Build history of the part. All positions in model axes, mm. Face numbers are marked on the shaded views. A direction names the side the tool comes from. Round coordinates to 2 decimals unless told otherwise and drop trailing zeros. Write each loop counter-clockwise with the first axis right and the second up, starting at its lowest first coordinate (ties: lowest second). Pieces come first, ordered by that corner, then holes. Notation, with made-up numbers: (-3.75, 23.5) - (11.25, 23.5) arc R22 ccw to (11.25, 42.5) - close; hole circle Ø11 at (-12.75, -8). An arc over 180 degrees is marked (long way). One line per question, with ' | ' between items.
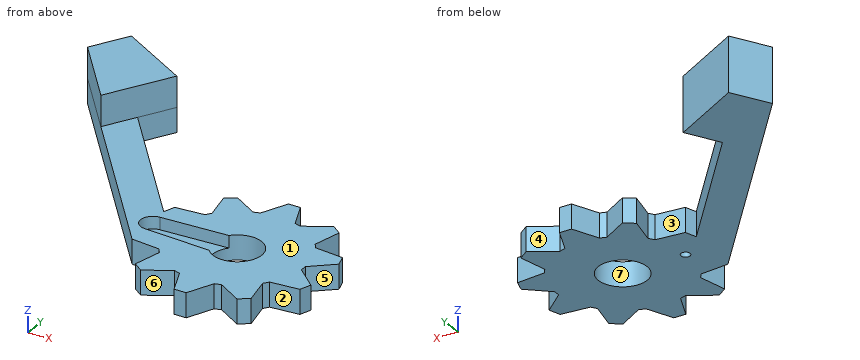
from build123d import *

# Parameters (mm, degrees)
SKETCH1_R           = 3.5
BOSS_EXTRUDE1_DEPTH = 4
BOSS_EXTRUDE2_DEPTH = 4
CUT_EXTRUDE1_DEPTH  = 2
SKETCH5_R           = 0.75
CUT_EXTRUDE2_DEPTH  = 59.571601855
SKETCH6_R           = 4
CUT_EXTRUDE3_DEPTH  = 10
BOSS_EXTRUDE3_DEPTH = 5


with BuildPart() as part:
    # Sketch1 → Boss-Extrude1 (new body)
    with BuildSketch(Plane.XY):
        with BuildLine():
            Line((-1, 15), (1, 15))
            Line((1, 15), (2.890622598, 10.613401952))
            ThreePointArc((2.890622598, 10.613401952), (3.399186938, 10.461621679), (3.899838338, 10.28548788))
            Line((3.899838338, 10.28548788), (8.00776179, 12.723040168))
            Line((8.00776179, 12.723040168), (9.625795779, 11.547469663))
            Line((9.625795779, 11.547469663), (8.57696395, 6.887357214))
            ThreePointArc((8.57696395, 6.887357214), (8.899186938, 6.465637775), (9.200693579, 6.02886703))
            Line((9.200693579, 6.02886703), (13.95683075, 5.586311432))
            Line((13.95683075, 5.586311432), (14.574864739, 3.684198399))
            Line((14.574864739, 3.684198399), (10.987196594, 0.530576113))
            ThreePointArc((10.987196594, 0.530576113), (11, 0), (10.987196594, -0.530576113))
            Line((10.987196594, -0.530576113), (14.574864739, -3.684198399))
            Line((14.574864739, -3.684198399), (13.95683075, -5.586311432))
            Line((13.95683075, -5.586311432), (9.200693579, -6.02886703))
            ThreePointArc((9.200693579, -6.02886703), (8.899186938, -6.465637775), (8.57696395, -6.887357214))
            Line((8.57696395, -6.887357214), (9.625795779, -11.547469663))
            Line((9.625795779, -11.547469663), (8.00776179, -12.723040168))
            Line((8.00776179, -12.723040168), (3.899838338, -10.28548788))
            ThreePointArc((3.899838338, -10.28548788), (3.399186938, -10.461621679), (2.890622598, -10.613401952))
            Line((2.890622598, -10.613401952), (1, -15))
            Line((1, -15), (-1, -15))
            Line((-1, -15), (-2.890622598, -10.613401952))
            ThreePointArc((-2.890622598, -10.613401952), (-3.399186938, -10.461621679), (-3.899838338, -10.28548788))
            Line((-3.899838338, -10.28548788), (-8.00776179, -12.723040168))
            Line((-8.00776179, -12.723040168), (-9.625795779, -11.547469663))
            Line((-9.625795779, -11.547469663), (-8.57696395, -6.887357214))
            ThreePointArc((-8.57696395, -6.887357214), (-8.899186938, -6.465637775), (-9.200693579, -6.02886703))
            Line((-9.200693579, -6.02886703), (-13.95683075, -5.586311432))
            Line((-13.95683075, -5.586311432), (-14.574864739, -3.684198399))
            Line((-14.574864739, -3.684198399), (-10.987196594, -0.530576113))
            ThreePointArc((-10.987196594, -0.530576113), (-11, 0), (-10.987196594, 0.530576113))
            Line((-10.987196594, 0.530576113), (-14.574864739, 3.684198399))
            Line((-14.574864739, 3.684198399), (-13.95683075, 5.586311432))
            Line((-13.95683075, 5.586311432), (-9.200693579, 6.02886703))
            ThreePointArc((-9.200693579, 6.02886703), (-8.899186938, 6.465637775), (-8.57696395, 6.887357214))
            Line((-8.57696395, 6.887357214), (-9.625795779, 11.547469663))
            Line((-9.625795779, 11.547469663), (-8.00776179, 12.723040168))
            Line((-8.00776179, 12.723040168), (-3.899838338, 10.28548788))
            ThreePointArc((-3.899838338, 10.28548788), (-3.399186938, 10.461621679), (-2.890622598, 10.613401952))
            Line((-2.890622598, 10.613401952), (-1, 15))
        make_face()
        Circle(SKETCH1_R, mode=Mode.SUBTRACT)
    extrude(amount=-BOSS_EXTRUDE1_DEPTH)

    # Sketch3 → Boss-Extrude2 (add)
    with BuildSketch(Plane.XY):
        Polygon((-41.373550062, 37.492275487), (-29.610808295, 30.834868856), (-32.690631554, 25.393235547), (-14.574864739, 3.684198399), (-10.987196594, 0.530576113), (-10.987196594, -0.530576113), (-14.574864739, -3.684198399), (-13.95683075, -5.586311432), (-44.821443781, 31.400311198), align=None)
    extrude(amount=-BOSS_EXTRUDE2_DEPTH)

    # Sketch4 → Cut-Extrude1 (cut)
    with BuildSketch(Plane.XY):
        with BuildLine():
            Line((-14.159121967, -1.99702088), (-2.291588247, -2.645491127))
            ThreePointArc((-2.291588247, -2.645491127), (-3.5, 0), (-2.291588247, 2.645491127))
            Line((-2.291588247, 2.645491127), (-14.159121967, 1.99702088))
            ThreePointArc((-14.159121967, 1.99702088), (-16.05, 0), (-14.159121967, -1.99702088))
        make_face()
    extrude(amount=-CUT_EXTRUDE1_DEPTH, mode=Mode.SUBTRACT)

    # Sketch5 → Cut-Extrude2 (cut, through all)
    with BuildSketch(Plane.XY):
        with Locations((-10.45, 0)):
            Circle(SKETCH5_R)
    extrude(amount=-CUT_EXTRUDE2_DEPTH, mode=Mode.SUBTRACT)

    # Sketch6 → Cut-Extrude3 (cut)
    with BuildSketch(Plane.XY):
        Circle(SKETCH6_R)
    extrude(amount=-CUT_EXTRUDE3_DEPTH, mode=Mode.SUBTRACT)

    # Sketch7 → Boss-Extrude3 (add)
    with BuildSketch(Plane.XY):
        Polygon((-29.610808295, 30.834868856), (-41.373550062, 37.492275487), (-44.821443781, 31.400311198), (-35.567281633, 20.310581908), align=None)
    extrude(amount=BOSS_EXTRUDE3_DEPTH)


solid = part.part
Q1. Saw through at B-B, the plane z = 1.5. List the corners of the cut face in (x, y).
Found:
outline: (-44.82, 31.4) - (-35.57, 20.31) - (-29.61, 30.83) - (-41.37, 37.49) - close
Q2. Pull direction X, two halves, no side cores. Call the marked faces 1, 2 and 3: +X half, -X half, draft (parallel to the pull), parting line (faces both ways), or undercut.
Found:
face 1: draft | face 2: +X half | face 3: undercut
Q3. Saw through at D-D, the plane x = -37.5. List the corners of the cut face in (y, z), then the cut area to 3 significant figures.
Found:
outline: (22.63, -4) - (35.3, -4) - (35.3, 5) - (22.63, 5) - close | area: 114 mm^2
Q4. Saw through at A-A, the plane x = -10.45. List the corners of the cut face in (y, z).
Found:
outline: (-5.91, -4) - (-0.75, -4) - (-0.75, -2) - (-2.2, -2) - (-2.2, 0) - (-5.91, 0) - close; (0.75, -4) - (5.91, -4) - (5.91, 0) - (2.2, 0) - (2.2, -2) - (0.75, -2) - close
Q5. Which spindle directions (+Z, -Z, +X, -X, +Y, -Y) get a long thin tool onto all of the face, cutting with end or side? Do the marked faces 4, 5, 6 and 7. Say none if no direction does.
Found:
face 4: +Z, -Z, +Y | face 5: +Z, -Z, +X | face 6: +Z, -Z, -Y | face 7: +Z, -Z
Q6. Drop flat-ended pins along their axis: pin 1 (1.6 mm diameter, centred on x = 0, z = -1, fed in from +Y); pin 2 (6 mm diameter, centred on x = -30, y = 28, fed in from -Z); pin 3 (2 mm diameter, centred on x = -14, y = -4.5, fed in from +Z); pin 4 (2 mm diameter, centred on x = -10, y = -0.5, fed in from +Z). Give the stop position or say it passes through.
Found:
pin 1: y = 15 | pin 2: z = -4 | pin 3: z = 0 | pin 4: z = -2
Q7. Saw through at C-C, the plane y = 23.5. List the corners of the cut face in (x, z), then the cut area to 3 significant figures.
Found:
outline: (-38.23, -4) - (-31.11, -4) - (-31.11, 0) - (-33.76, 0) - (-33.76, 5) - (-38.23, 5) - close | area: 50.8 mm^2
Q8. Drill centre lines: L1, parallel to Y at x = 0, z = -1.05; L2, parallel to Y at x = -10.45, z = -2.9; L3, parallel to Y at x = -8, z = -3.5. Where is each one in solid material? Low to high. Write a range as from..to.
Found:
L1: -15..-4, 4..15 | L2: -5.91..-0.75, 0.75..5.91 | L3: -12.72..12.72
